Check sheet for the modelled part. Datum: model origin and axes. Units: mm. A direction names the side the tool comes from. Give positions to 0.01 mm unless a question says otherwise; leave off trailing zeros. Loops run counter-clockwise (first coordinate to the right, second up) from the corner with the lowest first, then second, coordinate; pieces in that order, holes last. Notation, with made-up numbers: (33.25, -39) - (46.25, -39) arc R30 cw to (46.25, -5) - close; hole circle Ø11 at (30, 14). An arc over 180 degrees is marked (long way). Use one line per item in the form item = value.
from build123d import *

# Parameters (mm, degrees)
SKETCH_1_R          = 7.9
EXTRUDE_1_DEPTH     = 20
SKETCH_5_R          = 3.1
CUT_EXTRUDE_2_DEPTH = 20
SKETCH_6_R          = 10
EXTRUDE_2_DEPTH     = 2.5
SKETCH_7_R          = 3.5
CUT_EXTRUDE_3_DEPTH = 2.5
CHAMFER_1_SIZE      = 1


with BuildPart() as part:
    # 草图1 → 凸台-拉伸1 (new body)
    with BuildSketch(Plane(origin=(0, 0, 0), x_dir=(0, 0, -1), z_dir=(1, 0, 0))):
        Circle(SKETCH_1_R)
    extrude(amount=-EXTRUDE_1_DEPTH)

    # 草图5 → 切除-拉伸2 (cut, symmetric)
    with BuildSketch(Plane(origin=(0, 0, 0), x_dir=(1, 0, 0), z_dir=(0, 1, 0))):
        with Locations((-10, 0)):
            Circle(SKETCH_5_R)
    extrude(amount=CUT_EXTRUDE_2_DEPTH, both=True, mode=Mode.SUBTRACT)

    # 草图6 → 凸台-拉伸2 (add)
    with BuildSketch(Plane(origin=(0, 0, 0), x_dir=(0, 0, -1), z_dir=(1, 0, 0))):
        Circle(SKETCH_6_R)
    extrude(amount=EXTRUDE_2_DEPTH)

    # 草图7 → 切除-拉伸3 (cut)
    with BuildSketch(Plane(origin=(2.5, 0, 0), x_dir=(0, 0, -1), z_dir=(1, 0, 0))):
        Circle(SKETCH_7_R)
    extrude(amount=-CUT_EXTRUDE_3_DEPTH, mode=Mode.SUBTRACT)

    # 倒角1
    chamfer_1_edges = [part.edges().sort_by_distance(p)[0] for p in [
        (2.5, 0, 10),
    ]]
    chamfer(chamfer_1_edges, length=CHAMFER_1_SIZE)


solid = part.part
Item 1: Thickness scan on L1, parallel to X at y = 3.75, z = 0; L2, parallel to Y at x = -19, z = 0.25; L3, parallel to Y at x = 0.85, z = 0. Record the ranges inside material, lowest first.
Answer block:
L1 = -20 to -13.1, -6.9 to 2.5
L2 = -7.9 to 7.9
L3 = -10 to -3.5, 3.5 to 10
Item 2: Section check C-C on x = -10. Record the boundary of the cut face in (y, z).
Answer block:
outline = (-7.27, -3.1) arc R7.9 ccw to (7.27, -3.1) - close; (-7.27, 3.1) - (7.27, 3.1) arc R7.9 ccw to start
Item 3: Section check D-D on x = -14.5. Record the boundary of the cut face in (y, z).
Answer block:
outline = circle Ø15.8 at (0, 0)
Item 4: Section check A-A on z = 0. Record the boundary of the cut face in (x, y).
Answer block:
outline = (-20, -7.9) - (-13.1, -7.9) - (-13.1, 7.9) - (-20, 7.9) - close; (-6.9, -7.9) - (0, -7.9) - (0, -10) - (1.5, -10) - (2.5, -9) - (2.5, -3.5) - (0, -3.5) - (0, 3.5) - (2.5, 3.5) - (2.5, 9) - (1.5, 10) - (0, 10) - (0, 7.9) - (-6.9, 7.9) - close
Item 5: Access from +Z, -Z, +X, -X, +Y, -Y to the whole of each face (thin tool, end or side, straight path). Record for faces 4 (the face through (1.268, -1.341, -3.233)), 5 (the face through (2.5, -4, 0)), 6 (the face through (-9.86, 2.373, -7.535)).
Answer block:
face_4 = +X
face_5 = +Z, -Z, +X, +Y, -Y
face_6 = -X
Item 6: Gauge pin test, flat ends, axial feed: P1, Ø5, axis at x = -10, z = 0, coming from the -Y side; P2, Ø5, axis at y = -7, z = 6.5, coming from the -X side; P3, Ø5, axis at x = -8.5, y = 4.5, coming from the +Z side; P4, Ø2, axis at x = -13, z = 7.5, coming from the +Y side. Record the tip position at first contact, or that the pin passes through.
Answer block:
P1 = through
P2 = -20
P3 = 7.64
P4 = 4.49
Item 7: Mould release check, pull along Y, two halves, no side actions. Record for faces 1 (the face through (0, -4, -7)), 2 (the face through (0, 0, 0)), 3 (the face through (0.74, -9.76, 2.17)): released by +Y, released by -Y, zero draft, split by the parting line, or undercut.
Answer block:
face_1 = zero draft
face_2 = undercut
face_3 = split by the parting line
Item 8: Section check B-B on y = 0. Record the boundary of the cut face in (x, z).
Answer block:
outline = (-20, -7.9) - (0, -7.9) - (0, -10) - (1.5, -10) - (2.5, -9) - (2.5, -3.5) - (0, -3.5) - (0, 3.5) - (2.5, 3.5) - (2.5, 9) - (1.5, 10) - (0, 10) - (0, 7.9) - (-20, 7.9) - close; hole circle Ø6.2 at (-10, 0)
